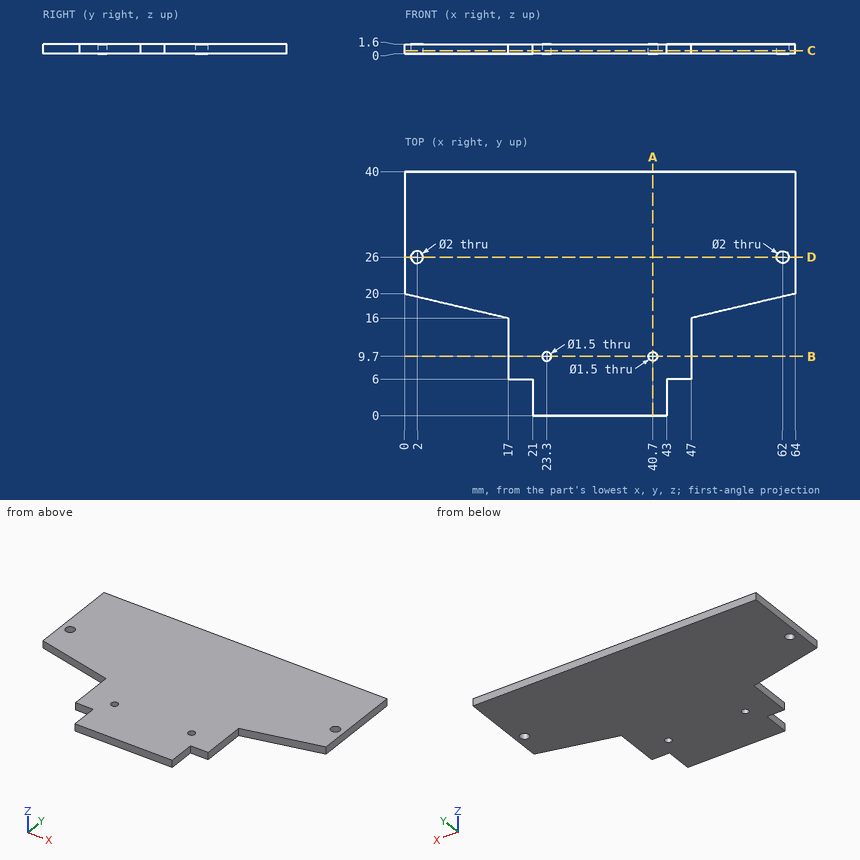
Study the drawing (mm; zero at the part's minimum x, y, z) and answer. Give positions to 0.01 mm unless a question says otherwise; leave off trailing zeros. Loops run counter-clockwise (first coordinate to the right, second up) from the corner with the lowest first, then second, coordinate; pieces in that order, holes last. Notation, with made-up numbers: (82.25, 27.5) - (126.25, 27.5) arc R19 cw to (126.25, 59.5) - close; hole circle Ø6 at (27.25, -27). An arc over 180 degrees is marked (long way). Use CSV: the item, a comma, the result in double quotes. Start each with the question number.
(1) Find section D-D, the plane y = 26. Determine the outline of the cut face in (x, z), plus the area to 3 significant figures.
(2) Find section C-C, the plane z = 0.5. Determine the outline of the cut face in (x, y), plus the area to 3 significant figures.
(3) Each of these flat-tipped pins is pushed along its axis until it touches: pin 1 (0.5 mm diameter, centred on y = 12.5, z = 1, fed in from -X); pin 2 (0.5 mm diameter, centred on x = 19.5, z = 0.5, fed in from -Y); pin 3 (0.8 mm diameter, centred on y = 10.5, z = 1, fed in from +X). Where does it stop, or does it pass through?
(4) Find the intervals of material crossed by L1, parallel to Y at x = 23.3, z = 0.9; L2, parallel to X at y = 3.5, z = 0.15; L3, parallel to X at y = 25.5, z = 0.2, in increasing order.
(5) Find section A-A, the plane x = 40.7. Determine the outline of the cut face in (y, z).
(6) Find section B-B, the plane y = 9.7. Determine the outline of the cut face in (x, z).
Results found:
1,outline,"(0, 0) - (1, 0) - (1, 1.6) - (0, 1.6) - close; (3, 0) - (61, 0) - (61, 1.6) - (3, 1.6) - close; (63, 0) - (64, 0) - (64, 1.6) - (63, 1.6) - close"
1,area,"96.0 mm^2"
2,outline,"(0, 20) - (17, 16) - (17, 6) - (21, 6) - (21, 0) - (43, 0) - (43, 6) - (47, 6) - (47, 16) - (64, 20) - (64, 40) - (0, 40) - close; hole circle Ø2 at (2, 26); hole circle Ø1.5 at (23.3, 9.7); hole circle Ø1.5 at (40.7, 9.7); hole circle Ø2 at (62, 26)"
2,area,"1,890 mm^2"
3,pin 1,"x = 17"
3,pin 2,"y = 6"
3,pin 3,"x = 47"
4,L1,"0 to 8.95, 10.45 to 40"
4,L2,"21 to 43"
4,L3,"0 to 1.13, 2.87 to 61.13, 62.87 to 64"
5,outline,"(0, 0) - (8.95, 0) - (8.95, 1.6) - (0, 1.6) - close; (10.45, 0) - (40, 0) - (40, 1.6) - (10.45, 1.6) - close"
6,outline,"(17, 0) - (22.55, 0) - (22.55, 1.6) - (17, 1.6) - close; (24.05, 0) - (39.95, 0) - (39.95, 1.6) - (24.05, 1.6) - close; (41.45, 0) - (47, 0) - (47, 1.6) - (41.45, 1.6) - close"
